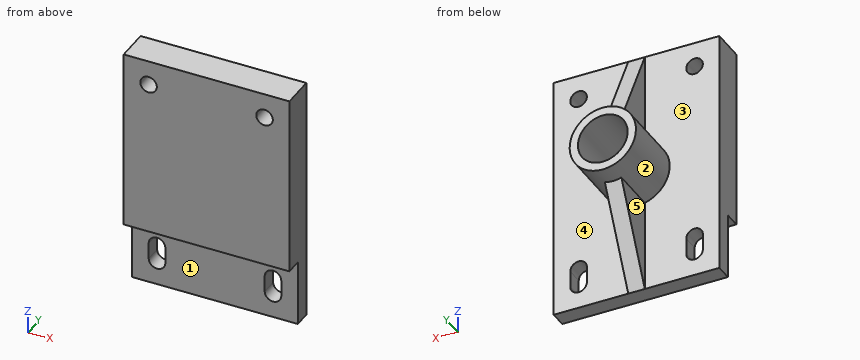
```python
from build123d import *

# Parameters (mm, degrees)
SKETCH_2_W          = 100
SKETCH_2_H          = 150
EXTRUDE_2_DEPTH     = 20
SKETCH_3_W          = 40
SKETCH_3_H          = 10
CUT_EXTRUDE_1_DEPTH = 127.589889012
SKETCH_5_R          = 5
CUT_EXTRUDE_3_DEPTH = 93.330926563
SKETCH_6_R          = 20
SKETCH_6_R_2        = 15
EXTRUDE_6_DEPTH     = 40
EXTRUDE_9_DEPTH     = 5
CUT_EXTRUDE_2_DEPTH = 99.615414617


with BuildPart() as part:
    # Эскиз2 → Бобышка-Вытянуть2 (new body)
    with BuildSketch(Plane(origin=(0, 0, 0), x_dir=(1, 0, 0), z_dir=(0, 1, 0))):
        Rectangle(SKETCH_2_W, SKETCH_2_H)
    extrude(amount=-EXTRUDE_2_DEPTH)

    # Эскиз3 → Вырез-Вытянуть1 (cut, through all)
    with BuildSketch(Plane(origin=(50, 0, 0), x_dir=(0, 0, -1), z_dir=(1, 0, 0))):
        with Locations((55, -15)):
            Rectangle(SKETCH_3_W, SKETCH_3_H)
    extrude(amount=-CUT_EXTRUDE_1_DEPTH, mode=Mode.SUBTRACT)

    # Эскиз5 → Вырез-Вытянуть3 (cut, through all)
    with BuildSketch(Plane(origin=(0, 0, 0), x_dir=(1, 0, 0), z_dir=(0, 1, 0))):
        with Locations(Location((-35, -60, 0), (0, 0, 270))):
            Circle(SKETCH_5_R)
        with BuildLine():
            Line((-30, 60), (-30, 50))
            ThreePointArc((-30, 50), (-35, 45), (-40, 50))
            Line((-40, 50), (-40, 60))
            ThreePointArc((-40, 60), (-35, 65), (-30, 60))
        make_face()
    cut_extrude_3 = extrude(amount=-CUT_EXTRUDE_3_DEPTH, mode=Mode.SUBTRACT)

    # Зеркальное отражение2: Вырез-Вытянуть3 across plane
    add(cut_extrude_3.mirror(Plane(origin=(0, 0, 0), x_dir=(0, 0, 1), z_dir=(1, 0, 0))), mode=Mode.SUBTRACT)

    # Эскиз6 → Бобышка-Вытянуть6 (add)
    with BuildSketch(Plane(origin=(0, 0, 0), x_dir=(1, 0, 0), z_dir=(0, 1, 0))):
        with Locations(Location((0, 0, 0), (0, 0, 90))):
            Circle(SKETCH_6_R)
        with Locations(Location((0, 0, 0), (0, 0, 270))):
            Circle(SKETCH_6_R_2, mode=Mode.SUBTRACT)
    extrude(amount=EXTRUDE_6_DEPTH)

    # Эскиз7 → Бобышка-Вытянуть9 (add, symmetric)
    with BuildSketch(Plane(origin=(0, 0, 0), x_dir=(0, 0, -1), z_dir=(1, 0, 0))):
        Polygon((-75, 0), (-15, 30), (-15, 0), align=None)
    extrude_9 = extrude(amount=EXTRUDE_9_DEPTH, both=True)

    # Зеркальное отражение3: Бобышка-Вытянуть9 across plane
    add(extrude_9.mirror(Plane.XY))

    # Эскиз4 → Вырез-Вытянуть2 (cut, through all)
    with BuildSketch(Plane(origin=(0, 0, 0), x_dir=(1, 0, 0), z_dir=(0, 1, 0))):
        with BuildLine():
            Line((-30, 60), (-30, 50))
            ThreePointArc((-30, 50), (-35, 45), (-40, 50))
            Line((-40, 50), (-40, 60))
            ThreePointArc((-40, 60), (-35, 65), (-30, 60))
        make_face()
    extrude(amount=-CUT_EXTRUDE_2_DEPTH, mode=Mode.SUBTRACT)


solid = part.part
```
Verification items for the finished model (mm, model axes). Face numbers are marked on the shaded views. A direction names the side the tool comes from. Give positions to 0.01 mm unless a question says otherwise; leave off trailing zeros. Write each loop counter-clockwise with the first axis right and the second up, starting at its lowest first coordinate (ties: lowest second). Pieces come first, ordered by that corner, then holes. Notation, with made-up numbers: (52.5, 77.25) - (84.5, 77.25) arc R6 ccw to (84.5, 87.25) - close; hole circle Ø10 at (59.5, 73.5). An arc over 180 degrees is marked (long way). Put each result on its own line as item: value.
Q1. Section check D-D on z = 46. Record the cut outline in (x, y).
Result:
outline: (-50, -20) - (50, -20) - (50, 0) - (5, 0) - (5, 14.5) - (-5, 14.5) - (-5, 0) - (-50, 0) - close
Q2. Depth check by flat-ended pin: P1, Ø4, axis at y = 11, z = 17.5, coming from the -X side; P2, Ø3, axis at x = 6, y = -14.5, coming from the -Z side; P3, Ø9, axis at x = -3.5, z = 5, coming from the +Y side. Enter the tip coordinate at first touch or a pass-through.
Result:
P1: x = -12.64
P2: z = -35
P3: y = 0
Q3. Section check B-B on x = -35. Record the cut outline in (y, z), and give its area (3 significant figures).
Result:
outline: (-20, -35) - (-10, -35) - (-10, -45) - (0, -45) - (0, 55) - (-20, 55) - close; (-20, 65) - (0, 65) - (0, 75) - (-20, 75) - close; (-10, -75) - (0, -75) - (0, -65) - (-10, -65) - close
area: 2,200 mm2
Q4. Section check C-C on y = -4.5. Record the cut outline in (x, z), and give its area (3 significant figures).
Result:
outline: (-50, -75) - (50, -75) - (50, 75) - (-50, 75) - close; hole (-40, -60) arc R5 ccw to (-30, -60) - (-30, -50) arc R5 ccw to (-40, -50) - close; hole circle Ø10 at (-35, 60); hole (30, -60) arc R5 ccw to (40, -60) - (40, -50) arc R5 ccw to (30, -50) - close; hole circle Ø10 at (35, 60)
area: 14,500 mm2
Q5. Section check A-A on z = -53. Record the cut outline in (x, y).
Result:
outline: (-50, -10) - (-40, -10) - (-40, 0) - (-50, 0) - close; (-30, -10) - (30, -10) - (30, 0) - (5, 0) - (5, 11) - (-5, 11) - (-5, 0) - (-30, 0) - close; (40, -10) - (50, -10) - (50, 0) - (40, 0) - close
Q6. Scan lines: probe 1 along Z at (x, y) = (35, -6.75); probe 2 along X at (y, z) = (19.5, 0); probe 3 along Z at (x, y) = (35, -11). Record each from-to range of solid material in increasing order. Write a range as from..to.
Result:
probe 1: -75..-65, -45..55, 65..75
probe 2: -20..-15, 15..20
probe 3: -35..55, 65..75
Q7. Set-up check for the marked faces 1, 2, 3, 4 and 5: record each of +Z, -Z, +X, -X, +Y, -Y from which the full face is reachable in a straight line by a thin tool's end or side.
Result:
face 1: -Z, +X, -X, -Y
face 2: +Y
face 3: -X, +Y
face 4: +X, +Y
face 5: -Z, -X, +Y
